Read the model definition and answer for the solid it produces. Units are mm, in the model's axes. Face numbers are marked on the shaded views. A direction names the side the tool comes from. Coordinates: 2 decimals unless noted, no trailing zeros. Write each loop counter-clockwise with the first axis right and the second up, starting at its lowest first coordinate (ties: lowest second). Pieces come first, ordered by that corner, then holes.
Item 1: Section B-B (y = 6) is taken. Give the vertices of the cut face in (x, z).
Item 2: Straight lines are drawn through the part: probe 1 along X at (y, z) = (26.8, -44); probe 2 along Y at (x, z) = (-29.5, -43); probe 3 along Z at (x, y) = (-24, 6.5). For each, find the intervals that lie inside material, in ascending order.
Item 3: Section D-D (x = 27.75) is taken. Give the vertices of the cut face in (y, z), then the cut area to 3 significant figures.
Item 4: Each of these flat-tipped pins is pushed along its axis until it touches: P1, Ø6, axis at x = -23.5, z = -24, coming from the +Y side; P2, Ø5, axis at x = -7.5, y = 18, coming from the -Z side; P3, Ø12, axis at x = 19, z = -16.5, coming from the -Y side; P4, Ø1.9, axis at x = -27.75, z = -44, coming from the +Y side. Where does it stop, or does it pass through?
Item 5: Section C-C (x = 16) is taken. Give the vertices of the cut face in (y, z), then the cut area to 3 significant figures.
Item 6: A tool of negligible diameter and unlimited length cuts with its end or side. For the marked faces 1 and 2, from which of +Z, -Z, +X, -X, +Y, -Y can it reach the whole face along a straight path? Write none if from no direction.
Item 7: Section A-A (z = -44) is taken. Give the vertices of the cut face in (x, y).
from build123d import *

# Parameters (mm, degrees)
BOSS_EXTRUDE1_DEPTH = 40
SKETCH2_R           = 1.6
CUT_EXTRUDE1_DEPTH  = 3
SKETCH3_W           = 80
SKETCH3_H           = 3
BOSS_EXTRUDE2_DEPTH = 8
SKETCH4_W           = 80
SKETCH4_H           = 0.830903327
CUT_EXTRUDE2_DEPTH  = 64.839370972
CHAMFER1_SIZE       = 5.693972562
CHAMFER1_SIZE_2     = 8
SKETCH5_R           = 1.6
CUT_EXTRUDE3_DEPTH  = 3


with BuildPart() as part:
    # Sketch1 → Boss-Extrude1 (new, symmetric)
    with BuildSketch(Plane(origin=(0, 0, 0), x_dir=(0, 0, -1), z_dir=(1, 0, 0))):
        Polygon((0, 0), (0, -4.242640687), (12.02081528, 7.778174593), (12.02081528, 3.538174593), (40, 25.757359313), (40, 29.58826264), (15.02081528, 9.751475936), (15.02081528, 15.02081528), align=None)
    extrude(amount=BOSS_EXTRUDE1_DEPTH, both=True)

    # Sketch2 → Cut-Extrude1 (cut)
    with BuildSketch(Plane(origin=(0, -2.121320344, -2.121320344), x_dir=(1, 0, 0), z_dir=(0, -0.7071067811865513, -0.7071067811865438))):
        with Locations(Location((-27.75, -2.75, 0), (0, 0, 270))):
            Circle(SKETCH2_R)
        with Locations(Location((27.75, -2.75, 0), (0, 0, 270))):
            Circle(SKETCH2_R)
    extrude(amount=-CUT_EXTRUDE1_DEPTH, mode=Mode.SUBTRACT)

    # Sketch3 → Boss-Extrude2 (add)
    with BuildSketch(Plane(origin=(0, 0, -40), x_dir=(-1, 0, 0), z_dir=(0, 0, -1))):
        with Locations((0, 27.257359313)):
            Rectangle(SKETCH3_W, SKETCH3_H)
    extrude(amount=BOSS_EXTRUDE2_DEPTH)

    # Sketch4 → Cut-Extrude2 (cut, through all)
    with BuildSketch(Plane(origin=(0, 0, -40), x_dir=(-1, 0, 0), z_dir=(0, 0, -1))):
        with Locations((0, 29.172810977)):
            Rectangle(SKETCH4_W, SKETCH4_H)
    extrude(amount=-CUT_EXTRUDE2_DEPTH, mode=Mode.SUBTRACT)

    # Chamfer1
    # the kernel refuses this chamfer: 8, 5.693972562 mm, written as the material it adds along each edge
    with BuildSketch(Plane(origin=(40, 9.751475936, -15.02081528), x_dir=(0, 0.9984646393058687, 0.05539281592229428), z_dir=(-1, 0, 0))) as chamfer1_piece_1_section:
        Polygon((CHAMFER1_SIZE * 0.998464639351, CHAMFER1_SIZE * 0.0553928159248), (CHAMFER1_SIZE_2 * 0.577556137161, CHAMFER1_SIZE_2 * 0.816350971352), (0, 0), align=None)
    chamfer1_piece_1 = extrude(amount=80, mode=Mode.PRIVATE)
    chamfer1_piece_1 = split(chamfer1_piece_1, bisect_by=Plane(origin=(0, 15.189171508, -15.189171508), z_dir=(0, -0.7071067811865511, -0.7071067811865441)), keep=Keep.TOP, mode=Mode.PRIVATE)
    add(chamfer1_piece_1)

    # Sketch5 → Cut-Extrude3 (cut)
    with BuildSketch(Plane.XZ.offset(-25.757359313)):
        with Locations(Location((-27.75, -44, 0), (0, 0, 270))):
            Circle(SKETCH5_R)
        with Locations(Location((27.75, -44, 0), (0, 0, 270))):
            Circle(SKETCH5_R)
    extrude(amount=-CUT_EXTRUDE3_DEPTH, mode=Mode.SUBTRACT)


solid = part.part
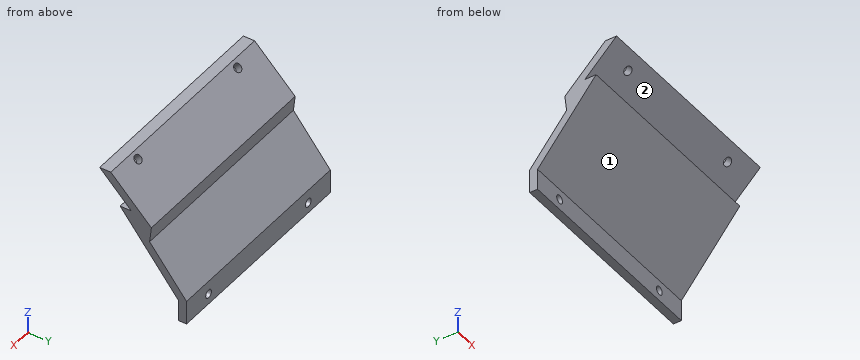
Established:
1. outline: (-40, -15.12) - (40, -15.12) - (40, -12.02) - (-40, -12.02) - close; (-40, -10.24) - (40, -10.24) - (40, -6) - (-40, -6) - close
2. probe 1: x = -40 to -29.35, -26.15 to 26.15, 29.35 to 40
2. probe 2: y = 25.76 to 28.76
2. probe 3: z = -15.75 to -12.02, -10.74 to -6.5
3. outline: (-4.24, 0) - (-1.31, -2.93) - (0.81, -0.81) - (0, 0) - close; (0.95, -5.2) - (7.78, -12.02) - (3.54, -12.02) - (25.76, -40) - (25.76, -42.4) - (28.76, -42.4) - (28.76, -38.95) - (14.73, -21.29) - (15.4, -15.4) - (3.08, -3.08) - close; (25.76, -48) - (28.76, -48) - (28.76, -45.6) - (25.76, -45.6) - close
3. area: 195 mm2
4. P1: stops at y = 19.26
4. P2: stops at z = -33.38
4. P3: stops at y = 3.54
4. P4: passes through
5. outline: (-4.24, 0) - (7.78, -12.02) - (3.54, -12.02) - (25.76, -40) - (25.76, -48) - (28.76, -48) - (28.76, -38.95) - (14.73, -21.29) - (15.4, -15.4) - (0, 0) - close
5. area: 214 mm2
6. face 1: -Z, +X, -X, -Y
6. face 2: +X, -X, -Y
7. outline: (-40, 25.76) - (-29.35, 25.76) - (-29.35, 28.76) - (-40, 28.76) - close; (-26.15, 25.76) - (26.15, 25.76) - (26.15, 28.76) - (-26.15, 28.76) - close; (29.35, 25.76) - (40, 25.76) - (40, 28.76) - (29.35, 28.76) - close
